from build123d import *

# Parameters (mm, degrees)
CROQUIS1_W                   = 5
CROQUIS1_H                   = 5.8
SALIENTE_EXTRUIR1_DEPTH      = 3.3
CROQUIS4_W                   = 1.1
CROQUIS4_H                   = 5.8
CORTAR_EXTRUIR1_DEPTH        = 1
CROQUIS5_W                   = 2.2
CROQUIS5_H                   = 0.9
SALIENTE_EXTRUIR2_DEPTH      = 8.1
REDONDEO4_R                  = 1
REDONDEO5_R                  = 1
SALIENTE_EXTRUIR3_DEPTH      = 4
SALIENTE_EXTRUIR3_DEPTH_BACK = 10
CROQUIS6_W                   = 0.6
CROQUIS6_H                   = 0.6


with BuildPart() as part:
    # Croquis1 → Saliente-Extruir1 (new body)
    with BuildSketch(Plane(origin=(0, 0, 0), x_dir=(1, 0, 0), z_dir=(0, 1, 0))):
        Rectangle(CROQUIS1_W, CROQUIS1_H)
    extrude(amount=SALIENTE_EXTRUIR1_DEPTH)

    # Croquis4 → Cortar-Extruir1 (cut)
    with BuildSketch(Plane.XZ):
        with Locations((-1.25, 0)):
            Rectangle(CROQUIS4_W, CROQUIS4_H)
        with Locations((1.25, 0)):
            Rectangle(CROQUIS4_W, CROQUIS4_H)
    extrude(amount=-CORTAR_EXTRUIR1_DEPTH, mode=Mode.SUBTRACT)

    # Croquis5 → Saliente-Extruir2 (add)
    with BuildSketch(Plane(origin=(0, 3.3, 0), x_dir=(1, 0, 0), z_dir=(0, 1, 0))):
        with Locations((0, 2.45)):
            Rectangle(CROQUIS5_W, CROQUIS5_H)
    extrude(amount=SALIENTE_EXTRUIR2_DEPTH)

    # Redondeo4
    redondeo4_edges = [part.edges().sort_by_distance(p)[0] for p in [
        (-1.1, 11.4, -2.45),
    ]]
    fillet(redondeo4_edges, radius=REDONDEO4_R)

    # Redondeo5
    redondeo5_edges = [part.edges().sort_by_distance(p)[0] for p in [
        (1.1, 11.4, -2.45),
    ]]
    fillet(redondeo5_edges, radius=REDONDEO5_R)

    # Croquis6 → Saliente-Extruir3 (add, two sides: drawn at the far end of the back side and taken through both)
    with BuildSketch(Plane.XZ.offset(-1).offset(-SALIENTE_EXTRUIR3_DEPTH_BACK)):
        with Locations((1.25, -0.3)):
            Rectangle(CROQUIS6_W, CROQUIS6_H)
        with Locations((-1.25, -0.3)):
            Rectangle(CROQUIS6_W, CROQUIS6_H)
    extrude(amount=SALIENTE_EXTRUIR3_DEPTH + SALIENTE_EXTRUIR3_DEPTH_BACK)


solid = part.part
Read the model definition and answer for the solid it produces. Units are mm, in the model's axes. A direction names the side the tool comes from. Round coordinates to 2 decimals unless told otherwise and drop trailing zeros. Order: outer loops, then holes, each group sorted by start corner. A loop starts at its lowest first (then second) coordinate and runs counter-clockwise, first axis right, second up. Notation, with made-up numbers: (50, 11.25) - (97, 11.25) arc R18 ccw to (97, 33.25) - close; hole circle Ø8 at (24, -29). An arc over 180 degrees is marked (long way). Use one line per item in the form item = value. Start each with the question number.
(1) The part is cut by section A-A (y = 4.25). Give the vertices of the cut face in (x, z), then the cut area to 3 significant figures.
(2) Flat-ended cylindrical pins translate along their axes: pin 1 Ø3 at (y, z) = (10, 2) entering from +X; pin 2 Ø0.5 at (y, z) = (-1, 0) entering from +X; pin 3 Ø0.7 at (x, y) = (1, 8.5) entering from +Z; pin 4 Ø1 at (y, z) = (7.5, -2.5) entering from +X. Find the tip coordinate at first contact, or state that the pin passes through.
(3) For faces 4 (the face through (-0.7, 0.5, 0)), 5 (the face through (-0.815, 11.099, -2.456)), 6 (the face through (1.1, 6.8, -2.4)), determine the directions among +Z, -Z, +X, -X, +Y, -Y from which every point of the face is accessible in a straight line to the end or side of a thin tool.
(4) Find the intervals of material crossed by line 1 along X through (y, z) = (0.5, -0.7); line 2 along X through (y, z) = (-1, -0.35); line 3 along Z through (x, y) = (-1, 8.5), in increasing order. Write a range as from..to.
(5) Determine the mould class of faces 1 (the face through (1.8, 0.5, 0)), 2 (the face through (0, 2, 2.9)), 3 (the face through (-1.1, 6.8, -2.4)) for opening direction X: +X half, -X half, draft (parallel to the pull), parting line (faces both ways), or undercut.
(6) The part is cut by section B-B (z = -1.05). Give the vertices of the cut face in (x, y).
(7) The part is cut by section C-C (y = 10.75). Give the vertices of the cut face in (x, z).
(8) The part is cut by section D-D (x = 0.4). Give the vertices of the cut face in (y, z).
Checked values:
q1.outline = (-1.55, -0.6) - (-0.95, -0.6) - (-0.95, 0) - (-1.55, 0) - close; (-1.1, -2.9) - (1.1, -2.9) - (1.1, -2) - (-1.1, -2) - close; (0.95, -0.6) - (1.55, -0.6) - (1.55, 0) - (0.95, 0) - close
q1.area = 2.70 mm^2
q2.pin_1 = through
q2.pin_2 = 1.55
q2.pin_3 = 0
q2.pin_4 = 1.1
q3.face_4 = +Z, -Z, -Y
q3.face_5 = -Z, -X, +Y
q3.face_6 = -Z, +X, +Y
q4.line_1 = -2.5..-1.8, -0.7..0.7, 1.8..2.5
q4.line_2 = -1.55..-0.95, 0.95..1.55
q4.line_3 = -2.9..-2, -0.6..0
q5.face_1 = undercut
q5.face_2 = draft
q5.face_3 = -X half
q6.outline = (-2.5, 0) - (-1.8, 0) - (-1.8, 1) - (-0.7, 1) - (-0.7, 0) - (0.7, 0) - (0.7, 1) - (1.8, 1) - (1.8, 0) - (2.5, 0) - (2.5, 3.3) - (-2.5, 3.3) - close
q7.outline = (-1.55, -0.6) - (-0.95, -0.6) - (-0.95, 0) - (-1.55, 0) - close; (-1.04, -2.9) - (1.04, -2.9) - (1.04, -2) - (-1.04, -2) - close; (0.95, -0.6) - (1.55, -0.6) - (1.55, 0) - (0.95, 0) - close
q8.outline = (0, -2.9) - (11.35, -2.9) - (11.35, -2) - (3.3, -2) - (3.3, 2.9) - (0, 2.9) - close
